```python
from build123d import *

# Parameters (mm, degrees)
F0_W     = 44
F0_H     = 40
F0_R     = 4.7625
F1_DEPTH = 3.175
F2_W     = 14.666667
F2_H     = 3.175
F3_DEPTH = 3.175


with BuildPart() as f1:
    # F0 (on Front) → F1 (new body)
    with BuildSketch(Plane.XZ):
        Rectangle(F0_W, F0_H)
        Circle(F0_R, mode=Mode.SUBTRACT)
    extrude(amount=F1_DEPTH)

    # F2 (on face) → F3 (join)
    with BuildSketch(Plane.XY.offset(20)):
        with Locations((-14.666666, -1.5875)):
            Rectangle(F2_W, F2_H)
        with Locations((14.666666, -1.5875)):
            Rectangle(F2_W, F2_H)
    extrude(amount=F3_DEPTH)


solid = f1.part
```
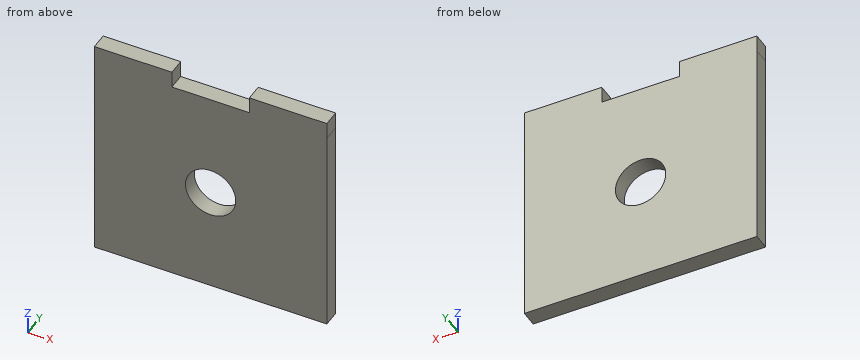
Here's how the part is built. I have some questions about the finished solid (model axes, mm). Coordinates: 2 decimals unless noted, no trailing zeros. Order: outer loops, then holes, each group sorted by start corner. A loop starts at its lowest first (then second) coordinate and runs counter-clockwise, first axis right, second up. Notation, with made-up numbers: (-24.75, -33.75) -> (-13.75, -33.75) arc R11 ccw to (-13.75, -23.75) -> close; hole circle Ø7 at (10, -28.75). An arc over 180 degrees is marked (long way). Return JSON: item names as keys, results as strings.
1) I'm going to push flat-ended pins straight in: P1, Ø5.5, axis at x = 0, z = 0, coming from the +Y side; P2, Ø1, axis at x = -3.5, y = -2, coming from the +Z side. Where does each tip first touch, or does it pass through?
Conclusion:
{"P1": "passes through", "P2": "stops at z = 20"}
2) If I drill on probe 1 along Z at (x, y) = (0, -1.1); probe 2 along X at (y, z) = (-0.75, -2); probe 3 along Z at (x, y) = (6.5, -0.35), over which ranges is the centre line in solid material (lowest first)?
Conclusion:
{"probe 1": "z = -20 to -4.76, 4.76 to 20", "probe 2": "x = -22 to -4.32, 4.32 to 22", "probe 3": "z = -20 to 20"}
3) If we section it at A-A on y = -1.2: List the corners of the cut face in (x, z) for me (1 decimal).
Conclusion:
{"outline": "(-22, -20) -> (22, -20) -> (22, 23.2) -> (7.3, 23.2) -> (7.3, 20) -> (-7.3, 20) -> (-7.3, 23.2) -> (-22, 23.2) -> close; hole circle Ø9.5 at (0, 0)"}
4) If we section it at C-C on x = 0: List the corners of the cut face in (y, z) for me (1 decimal), plus the area to 3 significant figures.
Conclusion:
{"outline": "(-3.2, -20) -> (0, -20) -> (0, -4.8) -> (-3.2, -4.8) -> close; (-3.2, 4.8) -> (0, 4.8) -> (0, 20) -> (-3.2, 20) -> close", "area": "96.8 mm²"}
5) If we section it at B-B on z = 0: List the corners of the cut face in (x, y) for me (1 decimal), plus the area to 3 significant figures.
Conclusion:
{"outline": "(-22, -3.2) -> (-4.8, -3.2) -> (-4.8, 0) -> (-22, 0) -> close; (4.8, -3.2) -> (22, -3.2) -> (22, 0) -> (4.8, 0) -> close", "area": "109 mm²"}
